For this review, take the finished solid that the model builds, in its own axes (mm). A direction names the side the tool comes from. Round coordinates to 2 decimals unless told otherwise and drop trailing zeros. Write each loop counter-clockwise with the first axis right and the second up, starting at its lowest first coordinate (ties: lowest second). Pieces come first, ordered by that corner, then holes. Notation, with made-up numbers: (27.5, 33) - (83.5, 33) arc R8 ccw to (83.5, 46) - close; hole circle Ø4 at (7, -33). An arc over 180 degrees is marked (long way). Answer in a Markdown table with one row per item. Add a question column.
from build123d import *

# Parameters (mm, degrees)
SKETCH1_W           = 109
SKETCH1_H           = 35
SKETCH1_R           = 2.1
BOSS_EXTRUDE1_DEPTH = 2
SKETCH2_W           = 92
SKETCH2_H           = 30
BOSS_EXTRUDE2_DEPTH = 2
SKETCH3_R           = 2.6
CUT_EXTRUDE1_DEPTH  = 127.925174808
CHAMFER1_SIZE       = 23
FILLET1_R           = 1.5


with BuildPart() as part:
    # Sketch1 → Boss-Extrude1 (new body)
    with BuildSketch(Plane(origin=(0, 0, 0), x_dir=(0, 0, -1), z_dir=(1, 0, 0))):
        with Locations((54.5, -17.5)):
            Rectangle(SKETCH1_W, SKETCH1_H)
        with Locations((104, -8.5)):
            Circle(SKETCH1_R, mode=Mode.SUBTRACT)
        with Locations(Location((104, -26.5, 0), (0, 0, 180))):
            Circle(SKETCH1_R, mode=Mode.SUBTRACT)
        with Locations((80, -26.5)):
            Circle(SKETCH1_R, mode=Mode.SUBTRACT)
        with Locations(Location((80, -8.5, 0), (0, 0, 180))):
            Circle(SKETCH1_R, mode=Mode.SUBTRACT)
        with Locations((5, -26.5)):
            Circle(SKETCH1_R, mode=Mode.SUBTRACT)
        with Locations(Location((5, -8.5, 0), (0, 0, 180))):
            Circle(SKETCH1_R, mode=Mode.SUBTRACT)
        with Locations(Location((29, -26.5, 0), (0, 0, 180))):
            Circle(SKETCH1_R, mode=Mode.SUBTRACT)
        with Locations((29, -8.5)):
            Circle(SKETCH1_R, mode=Mode.SUBTRACT)
    extrude(amount=BOSS_EXTRUDE1_DEPTH)

    # Sketch2 → Boss-Extrude2 (add)
    with BuildSketch(Plane(origin=(2, 0, 0), x_dir=(0, 0, -1), z_dir=(1, 0, 0))):
        with Locations((54.5, -50)):
            Rectangle(SKETCH2_W, SKETCH2_H)
    extrude(amount=-BOSS_EXTRUDE2_DEPTH)

    # Sketch3 → Cut-Extrude1 (cut, through all)
    with BuildSketch(Plane(origin=(2, 0, 0), x_dir=(0, 0, -1), z_dir=(1, 0, 0))):
        with Locations((13.7, -50)):
            Circle(SKETCH3_R)
        with Locations((39.5, -50)):
            Circle(SKETCH3_R)
        with Locations(Location((95.3, -50, 0), (0, 0, 180))):
            Circle(SKETCH3_R)
        with Locations(Location((69.5, -50, 0), (0, 0, 180))):
            Circle(SKETCH3_R)
        with Locations((69.5, -18)):
            Circle(SKETCH3_R)
        with Locations(Location((39.5, -18, 0), (0, 0, 180))):
            Circle(SKETCH3_R)
    extrude(amount=-CUT_EXTRUDE1_DEPTH, mode=Mode.SUBTRACT)

    # Chamfer1
    # the kernel refuses this chamfer: 23 mm, written as the material it adds along each edge
    with BuildSketch(Plane(origin=(2, -35, -100.5), x_dir=(0, 0.027495876610586077, -0.9996219169112968), z_dir=(-1, 0, 0))) as chamfer1_piece_1_section:
        Polygon((CHAMFER1_SIZE * 0.999621916911, CHAMFER1_SIZE * 0.0274958766106), (-CHAMFER1_SIZE * 0.0274958766106, CHAMFER1_SIZE * 0.999621916911), (0, 0), align=None)
    chamfer1_piece_1 = extrude(amount=2, mode=Mode.PRIVATE)
    chamfer1_piece_1 = split(chamfer1_piece_1, bisect_by=Plane(origin=(1, -44.672301489, -109), z_dir=(0, 0, 1)), keep=Keep.TOP, mode=Mode.PRIVATE)
    add(chamfer1_piece_1)
    with BuildSketch(Plane(origin=(2, -35, -8.5), x_dir=(0, 0.02749587661058667, 0.9996219169112968), z_dir=(-1, 0, 0))) as chamfer1_piece_2_section:
        Polygon((CHAMFER1_SIZE * 0.999621916911, -CHAMFER1_SIZE * 0.0274958766106), (-CHAMFER1_SIZE * 0.0274958766106, -CHAMFER1_SIZE * 0.999621916911), (0, 0), align=None)
    chamfer1_piece_2 = extrude(amount=2, mode=Mode.PRIVATE)
    chamfer1_piece_2 = split(chamfer1_piece_2, bisect_by=Plane(origin=(1, -44.672301489, 0), z_dir=(0, 0, -1)), keep=Keep.TOP, mode=Mode.PRIVATE)
    add(chamfer1_piece_2)

    # Fillet1
    fillet1_edges = [part.edges().sort_by_distance(p)[0] for p in [
        (1, -65, -8.5),
        (1, -65, -100.5),
        (1, 0, 0),
        (1, 0, -109),
        (1, -58, -8.5),
        (1, -58, -100.5),
        (1, -49.5, 0),
        (1, -49.5, -109),
    ]]
    fillet(fillet1_edges, radius=FILLET1_R)


solid = part.part
Q1. Draft analysis for pull direction Z (two halves, no side actions). For faces 1 (the face through (1, -53.7, -104.8)), 2 (the face through (1, -61, -8.5)), 3 (the face through (0.99, -26.59, -106.1)), 4 (the face through (1.01, -52.54, -13.14)), state which applies: released by +Z, released by -Z, zero draft, split by the parting line, or undercut.
Q2. Add section C-C on y = -26.5. State the section outline as (x, z) points.
Q3. Insertion check: pin 1 Ø2.5 at (y, z) = (-26.5, -5) entering from -X. The pin has a flat end and moves straight along its axis. Give the tip position at first contact, or say it passes through.
Q4. To check wall thickness, follow probe 1 along Y at (x, z) = (0.5, -29); probe 2 along Y at (x, z) = (0.9, -69.5); probe 3 along Y at (x, z) = (0.25, -95.5). State the ranges of each line that lie inside material, in increasing order.
Q5. Tool access review of faces 5 (the face through (1.014, -51.582, -37.437)), 6 (the face through (1, -61, -100.5)): name each direction out of +Z, -Z, +X, -X, +Y, -Y from which nothing blocks a thin tool from reaching the whole face with its end or side.
Q6. Add section B-B on x = 1. Count the separate pieces of the cut face and the enclosed holes in it, then the cut area to 3 significant figures.
Q7. Add section D-D on z = -39.5. State the section outline as (x, y) points.
Q8. Add section A-A on z = -13.7. State the section outline as (x, y) points.
Answer sheet:
| question | item | result |
|---|---|---|
| 1 | face 1 | released by -Z |
| 1 | face 2 | released by +Z |
| 1 | face 3 | undercut |
| 1 | face 4 | undercut |
| 2 | outline | (0, -109) - (2, -109) - (2, -106.1) - (0, -106.1) - close; (0, -101.9) - (2, -101.9) - (2, -82.1) - (0, -82.1) - close; (0, -77.9) - (2, -77.9) - (2, -31.1) - (0, -31.1) - close; (0, -26.9) - (2, -26.9) - (2, -7.1) - (0, -7.1) - close; (0, -2.9) - (2, -2.9) - (2, 0) - (0, 0) - close |
| 3 | pin 1 | passes through |
| 4 | probe 1 | y = -65 to -28.6, -24.4 to -10.6, -6.4 to 0 |
| 4 | probe 2 | y = -65 to -52.6, -47.4 to -20.6, -15.4 to 0 |
| 4 | probe 3 | y = -65 to -52.59, -47.41 to 0 |
| 5 | face 5 | +X, -X |
| 5 | face 6 | -Z, +X, -X, -Y |
| 6 | separate pieces | 1 |
| 6 | enclosed holes | 14 |
| 6 | area | 6,650 mm² |
| 7 | outline | (0, -65) - (2, -65) - (2, -52.6) - (0, -52.6) - close; (0, -47.4) - (2, -47.4) - (2, -20.6) - (0, -20.6) - close; (0, -15.4) - (2, -15.4) - (2, 0) - (0, 0) - close |
| 8 | outline | (0, -65) - (2, -65) - (2, -52.6) - (0, -52.6) - close; (0, -47.4) - (2, -47.4) - (2, 0) - (0, 0) - close |
